Source: CAD feature listing. Evaluate the final solid. Frame: model axes, mm. Round coordinates to 2 decimals unless told otherwise and drop trailing zeros. Order: outer loops, then holes, each group sorted by start corner. A loop starts at its lowest first (then second) coordinate and runs counter-clockwise, first axis right, second up. Notation, with made-up numbers: M 61.5,-31 L 110.5,-31 A17 ccw 110.5,2 Z; hole C 13.5,-17.75 d7. An arc over 180 degrees is marked long. Answer as CSV lines item,"result". Start each with the question number.
Item 1: Pull-direction query (X, two-part tool) for faces 1 (the face through (-15.564, -8.674, 0.038)), 2 (the face through (-6, 9, 10)), 3 (the face through (-9.76, 0.11, -2.17)), 4 (the face through (7.749, 8.674, -13.498)); classes: +X half, -X half, draft (parallel to the pull), parting line (faces both ways), or undercut.
Item 2: First-contact query: P1, Ø5, axis at x = 12, y = -2, coming from the +Z side; P2, Ø8, axis at y = -2.5, z = 1, coming from the +X side. Flat tips, straight axial feed; report the tip coordinate or a pass-through.
Item 3: Section query A-A on y = 1.25. Return the cut outline in (x, z), plus the area to 3 significant figures.
Item 4: Line query: line 1 (X direction, y = 4.25, z = 0); line 2 (Z direction, x = -0.5, y = 5.75); line 3 (Z direction, x = -2, y = -2.75). Output: solid intervals per line, ascending. Write a range as [from, to].
from build123d import *

# Parameters (mm, degrees)
EXTRUDE_1_DEPTH     = 9
SKETCH_2_R          = 10
CUT_EXTRUDE_1_DEPTH = 30.137604569
CHAMFER_1_SIZE      = 1.2


with BuildPart() as part:
    # 草图1 → 凸台-拉伸1 (new, symmetric)
    with BuildSketch(Plane(origin=(0, 0, 0), x_dir=(1, 0, 0), z_dir=(0, 1, 0))):
        Polygon((17.320508076, 0), (8.660254038, 15), (-8.660254038, 15), (-17.320508076, 0), (-8.660254038, -15), (8.660254038, -15), align=None)
    extrude(amount=EXTRUDE_1_DEPTH, both=True)

    # 草图2 → 切除-拉伸1 (cut, through all)
    with BuildSketch(Plane(origin=(0, 9, 0), x_dir=(1, 0, 0), z_dir=(0, 1, 0))):
        with Locations(Location((0, 0, 0), (0, 0, 270))):
            Circle(SKETCH_2_R)
    extrude(amount=-CUT_EXTRUDE_1_DEPTH, mode=Mode.SUBTRACT)

    # 倒角1
    chamfer_1_edges = [part.edges().sort_by_distance(p)[0] for p in [
        (0, -9, -10),
        (0, 9, -10),
    ]]
    chamfer(chamfer_1_edges, length=CHAMFER_1_SIZE)

    # 草图3 → 切除-旋转1 (revolve, cut)
    with BuildSketch(Plane.XY, mode=Mode.PRIVATE) as cut_revolve_1_sk:
        Polygon((17.320508076, 9), (15, 9), (17.320508076, 7.660254038), align=None)
    cut_revolve_1 = revolve(cut_revolve_1_sk.sketch.rotate(Axis((0, 9, 0), (0, -1, 0)), 270), axis=Axis((0, 9, 0), (0, -1, 0)), mode=Mode.SUBTRACT)

    # 镜向1: 切除-旋转1 across plane
    add(cut_revolve_1.mirror(Plane.ZX), mode=Mode.SUBTRACT)


solid = part.part
Results:
1,face 1,"-X half"
1,face 2,"draft"
1,face 3,"undercut"
1,face 4,"+X half"
2,P1,"z = 13.55"
2,P2,"x = 17.32"
3,outline,"M -17.32,0 L -8.66,-15 L 8.66,-15 L 17.32,0 L 8.66,15 L -8.66,15 Z; hole C 0,0 d20"
3,area,"465 mm^2"
4,line 1,"[-17.32, -10], [10, 17.32]"
4,line 2,"[-15, -9.99], [9.99, 15]"
4,line 3,"[-15, -9.8], [9.8, 15]"
